Can you work these out from the model? Positions are in its coordinate system, mm. Face numbers are marked on the shaded views. A direction names the side the tool comes from. Round coordinates to 2 decimals unless told otherwise and drop trailing zeros. Write each loop counter-clockwise with the first axis right and the second up, starting at its lowest first coordinate (ties: lowest second). Pieces come first, ordered by that corner, then holes. Notation, with made-up numbers: M -16,23 L 9,23 A20 cw 9,47 Z; hole C 68.25,30 d1. An arc over 180 degrees is marked long. Answer in a Markdown table with one row per item. Add a question column.
(1) If we mould it in two halves opening along X, with no side actions, what happens to the marked faces 1, 2 and 3? For each: released by +X, released by -X, zero draft, split by the parting line, or undercut.
(2) Suppose I cut it at B-B, the plane y = 15. Write out the boundary of the cut face in (x, z), then the cut area to 3 significant figures.
(3) I'm going to push flat-ended pins straight in: pin 1 (2.5 mm diameter, centred on y = 16, z = 31.5, fed in from -X); pin 2 (5 mm diameter, centred on y = 10, z = 34, fed in from +X); pin 3 (15 mm diameter, centred on x = 30, y = 21, fed in from +Z). Where does each tip first touch, or does it pass through?
(4) For the marked faces 4, 5, 6, 7 and 8, which set-ups out of +Z, -Z, +X, -X, +Y, -Y let a thin tool reach every point of the face, with its end or its side?
(5) If I drill on probe 1 along Y at (x, z) = (-40.5, -25); probe 2 along Z at (x, y) = (-37, 2.5); probe 3 along Z at (x, y) = (33, 7.5), over which ranges is the centre line in solid material (lowest first)?
(6) Suppose I cut it at D-D, the plane y = 7. Write out the boundary of the cut face in (x, z), then the cut area to 3 significant figures.
(7) Suppose I cut it at A-A, the plane x = 0. Write out the boundary of the cut face in (y, z), then the cut area to 3 significant figures.
(8) Suppose I cut it at C-C, the plane z = 0. Write out the boundary of the cut face in (x, y), then the cut area to 3 significant figures.
Autodesk Fusion 360 part; units mm, degrees
sketch "Sketch1" plane through (0, 0, 0) normal (0, 1, 0) x (1, 0, 0)
  line L0 (-50, -30) -> (50, -30)
  line L1 (50, -30) -> (50, 30)
  line L2 (50, 30) -> (-50, 30)
  line L3 (-50, 30) -> (-50, -30)
  dimension "d1" = 100
  dimension "d2" = 60
extrude "Extrude1" add sketch "Sketch1" along normal blind 30
sketch "Sketch2" plane through (0, 0, 0) normal (0, -1, 0) x (1, 0, 0)
  line L0 (-50, 30) -> (-50, -30)
  line L1 (-50, -30) -> (50, -30)
  line L2 (50, -30) -> (50, 30)
  line L3 (50, 30) -> (-50, 30)
  circle A0 centre (0, 0) radius 25
  dimension "d5" = 50
extrude "Extrude2" add sketch "Sketch2" along normal blind 20 contours A0
sketch "Sketch3" plane through (0, 0, 30) normal (0, 0, 1) x (-1, 0, 0)
  line L0 (50, 0) -> (-50, 0)
  line L1 (-50, 0) -> (-50, -30)
  line L2 (-50, -30) -> (50, -30)
  line L3 (50, -30) -> (50, 0)
  circle A0 centre (-35, -15) radius 10
  dimension "d8" = 20
  dimension "d9" = 15
extrude "Extrude3" add sketch "Sketch3" along normal blind 5 contours A0
sketch "Sketch4" plane through (0, 0, 30) normal (0, 0, 1) x (-1, 0, 0)
  circle A0 centre (-35, -15) radius 10
  line L0 (50, 0) -> (-50, 0)
  line L1 (-50, 0) -> (-50, -30)
  line L2 (-50, -30) -> (50, -30)
  line L3 (50, -30) -> (50, 0)
sketch "Sketch5" plane through (0, 0, 30) normal (0, 0, 1) x (-1, 0, 0)
  line L0 (-20, 0) -> (10, 0)
  line L1 (10, 0) -> (10, -30)
  line L2 (10, -30) -> (-20, -30)
  line L3 (-20, -30) -> (-20, 0)
  line L4 (-20, 0) -> (-10, -10)
  line L5 (10, 0) -> (25, 0)
  dimension "d12" = 30
extrude "Extrude4" add sketch "Sketch5" along normal blind 10
sketch "Sketch6" plane through (0, 0, 30) normal (0, 0, 1) x (-1, 0, 0)
  line L0 (-20, 0) -> (-10, -10)
  line L1 (35, -10) -> (45, -10)
  line L2 (45, -10) -> (45, -20)
  line L3 (45, -20) -> (35, -20)
  line L4 (35, -20) -> (35, -10)
  line L5 (35, -10) -> (45, -20) construction
  line L6 (45, -10) -> (35, -20) construction
  line L7 (50, -30) -> (50, 0)
  point P0 (40, -15)
  dimension "d15" = 15
extrude "Extrude5" add sketch "Sketch6" along normal blind 5
sketch "Sketch7" plane through (0, 0, 30) normal (0, 0, 1) x (-1, 0, 0)
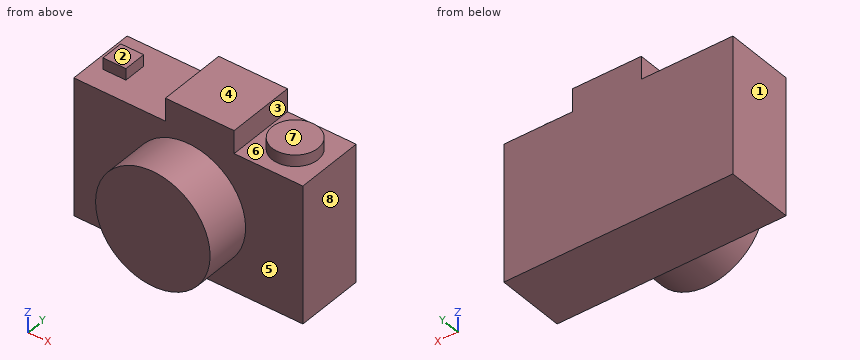
Calculated:
| question | item | result |
|---|---|---|
| 1 | face 1 | released by -X |
| 1 | face 2 | zero draft |
| 1 | face 3 | undercut |
| 2 | outline | M -50,-30 L 50,-30 L 50,30 L 45,30 L 45,35 L 25,35 L 25,30 L 20,30 L 20,40 L -10,40 L -10,30 L -35,30 L -35,35 L -45,35 L -45,30 L -50,30 Z |
| 2 | area | 6,450 mm² |
| 3 | pin 1 | x = -45 |
| 3 | pin 2 | x = 44.68 |
| 3 | pin 3 | z = 35 |
| 4 | face 4 | +Z, +X, -X, +Y, -Y |
| 4 | face 5 | -Y |
| 4 | face 6 | +Z |
| 4 | face 7 | +Z, +X, +Y, -Y |
| 4 | face 8 | +Z, -Z, +X, +Y, -Y |
| 5 | probe 1 | 0 to 30 |
| 5 | probe 2 | -30 to 30 |
| 5 | probe 3 | -30 to 35 |
| 6 | outline | M -50,-30 L 50,-30 L 50,30 L 41,30 L 41,35 L 29,35 L 29,30 L 20,30 L 20,40 L -10,40 L -10,30 L -50,30 Z |
| 6 | area | 6,360 mm² |
| 7 | outline | M -20,-25 L 0,-25 L 0,-30 L 30,-30 L 30,40 L 0,40 L 0,25 L -20,25 Z |
| 7 | area | 3,100 mm² |
| 8 | outline | M -50,0 L -25,0 L -25,-20 L 25,-20 L 25,0 L 50,0 L 50,30 L -50,30 Z |
| 8 | area | 4,000 mm² |
